Autodesk Inventor part; units mm, degrees
ref_plane "YZ Plane" through (0, 0, 0) normal (1, 0, 0) x (0, 1, 0)
ref_plane "XZ Plane" through (0, 0, 0) normal (0, 1, 0) x (-1, 0, 0)
ref_plane "XY Plane" through (0, 0, 0) normal (0, 0, 1) x (1, 0, 0)
sketch "Sketch1" plane through (0, 0, 0) normal (0, 0, 1) x (1, 0, 0)
  line L0 (0, 0) -> (0, 33.02)
  line L1 (0, 33.02) -> (203.2, 33.02)
  line L2 (203.2, 33.02) -> (203.2, 0)
  line L3 (203.2, 0) -> (0, 0)
  dimension "d0" = 203.2
  dimension "d1" = 33.02
extrude "Extrusion1" add sketch "Sketch1" along normal blind 190.5
sketch "Sketch2" plane through (0, 33.02, 0) normal (0, 1, 0) x (1, 0, 0)
  line L0 (196.85, -184.15) -> (6.35, -184.15)
  line L1 (6.35, -184.15) -> (6.35, -6.35)
  line L2 (6.35, -6.35) -> (196.85, -6.35)
  line L3 (196.85, -6.35) -> (196.85, -184.15)
  line L4 (203.2, 0) -> (203.2, -190.5)
  line L5 (203.2, 0) -> (0, 0)
  line L6 (0, 0) -> (0, -190.5)
  dimension "d4" = 190.5
  dimension "d5" = 177.8
  dimension "d6" = 6.35
  dimension "d7" = 6.35
extrude "Extrusion2" cut sketch "Sketch2" against normal blind 11.43
sketch "Sketch3" plane through (203.2, 0, 0) normal (1, 0, 0) x (0, 0, -1)
  line L0 (-6.35, 21.59) -> (-184.15, 21.59)
  line L1 (0, 33.02) -> (-190.5, 33.02)
  line L2 (-26.7226, 33.02) -> (-26.7226, 21.59)
  line L3 (-6.35, 21.59) -> (-6.35, 33.02)
  line L4 (-26.7226, 33.02) -> (-6.35, 33.02)
  point P0 (0, 0)
extrude "Extrusion3" cut sketch "Sketch3" against normal blind 11.43
properties part number "Photosynthetic_Wind_Base"
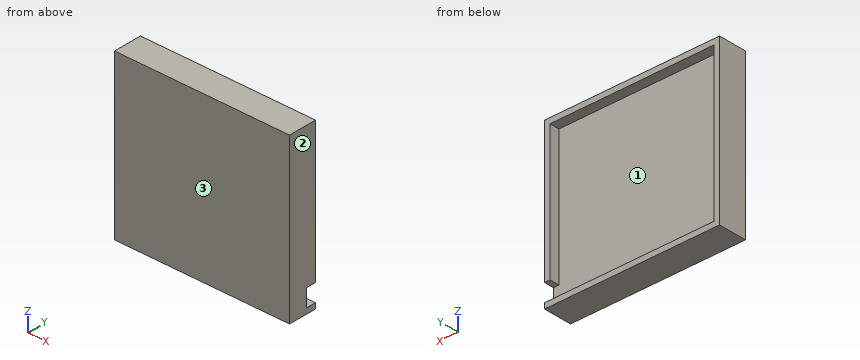
Model file for the job. Use its own axes, mm. Face numbers are marked on the shaded views. Round coordinates to 2 decimals unless told otherwise and drop trailing zeros. Order: outer loops, then holes, each group sorted by start corner. A loop starts at its lowest first (then second) coordinate and runs counter-clockwise, first axis right, second up.
(1) Band-saw the part on B-B (z = 172). List the corners of the cut face in (x, y), then the cut area to 3 significant figures.
(2) Drill centre lines: line 1 (X direction, y = 25.5, z = 161); line 2 (Z direction, x = 186, y = 25); line 3 (Y direction, x = 191, z = 90). Where is each one in solid material? Low to high.
(3) Band-saw the part on C-C (z = 17). List the corners of the cut face in (x, y), then the cut area to 3 significant figures.
(4) Band-saw the part on A-A (x = 86). List the corners of the cut face in (y, z).
(5) Pin check, flat tips, straight feed: pin 1 (10 mm diameter, centred on y = 25, z = 49.5, fed in from -X); pin 2 (6 mm diameter, centred on x = 80, z = 164.5, fed in from +Y). Stop position of each tip, or through.
(6) Pull direction X, two halves, no side cores. Call the marked faces 1, 2 and 3: released by +X, released by -X, zero draft, split by the parting line, or undercut.
Verdict:
1. outline: (0, 0) - (203.2, 0) - (203.2, 33.02) - (196.85, 33.02) - (196.85, 21.59) - (6.35, 21.59) - (6.35, 33.02) - (0, 33.02) - close
1. area: 4,530 mm2
2. line 1: x = 0 to 6.35, 196.85 to 203.2
2. line 2: z = 0 to 6.35, 184.15 to 190.5
2. line 3: y = 0 to 21.59
3. outline: (0, 0) - (203.2, 0) - (203.2, 21.59) - (6.35, 21.59) - (6.35, 33.02) - (0, 33.02) - close
3. area: 4,460 mm2
4. outline: (0, 0) - (33.02, 0) - (33.02, 6.35) - (21.59, 6.35) - (21.59, 184.15) - (33.02, 184.15) - (33.02, 190.5) - (0, 190.5) - close
5. pin 1: stops at x = 0
5. pin 2: stops at y = 21.59
6. face 1: undercut
6. face 2: released by +X
6. face 3: zero draft
